Input: part model. Units: mm. Frame: model coordinates. A direction names the side the tool comes from. Coordinates: 2 decimals unless noted, no trailing zeros. Write each loop counter-clockwise with the first axis right and the second up, starting at its lowest first coordinate (ties: lowest second). Pieces come first, ordered by that corner, then holes. Notation, with made-up numbers: (-2.5, 38.25) - (15.5, 38.25) arc R3 cw to (15.5, 43.25) - close; hole circle Ø7 at (45, -20). An arc over 180 degrees is marked (long way). Put each result on its own line as item: value. Start each with the question number.
1. Cut plane A-A, the plane z = -32. Return loops of the section in (x, y), and give its area (3 significant figures).
2. Access query for faces 4 (the cylindrical face through (-8, -48, -8)), 5 (the flat face through (-153, 5, -58)), 6 (the flat face through (-200, 2, -61)), 7 (the cylindrical face through (-101, -48, -64)). Directions: +Z, -Z, +X, -X, +Y, -Y. A direction counts if a zero-diameter tool reaches every point of the face in a straight line with its end or side. Return the directions, or none.
3. Line query: line 1 (X direction, y = 2, z = -4); line 2 (X direction, y = 3, z = -62); line 3 (Z direction, x = -189, y = -51). Output: solid intervals per line, ascending.
4. Pull-direction query (Z, two-part tool) for faces 1 (the flat face through (-110, 3, -27)), 2 (the flat face through (-97, -27, -67)), 3 (the flat face through (-197, 4.5, -61)); classes: released by +Z, released by -Z, zero draft, split by the parting line, or undercut.
5. Cut plane C-C, the plane x = -164. Return loops of the section in (y, z), and give its area (3 significant figures).
6. Pin query (flat end, axial travel): pin 1 (1.5 mm diameter, centred on y = -27, z = -65, fed in from +X); pin 2 (2 mm diameter, centred on y = 4.5, z = -36.5, fed in from -X); pin 3 (3.5 mm diameter, centred on x = -178.5, y = 1.5, fed in from +Z); pin 4 (1.5 mm diameter, centred on y = -6.5, z = -67.5, fed in from -X). Return the tip coordinate at first contact, or that it passes through.
7. Cut plane B-B, the plane y = -48. Return loops of the section in (x, z), and give its area (3 significant figures).
Autodesk Inventor part; units mm, degrees
ref_plane "YZ Plane" through (0, 0, 0) normal (1, 0, 0) x (0, 1, 0)
ref_plane "XZ Plane" through (0, 0, 0) normal (0, 1, 0) x (-1, 0, 0)
ref_plane "XY Plane" through (0, 0, 0) normal (0, 0, 1) x (1, 0, 0)
sketch "スケッチ1" plane through (0, 0, 0) normal (0, 1, 0) x (-1, 0, 0)
  line L0 (0, 0) -> (204, 0)
  line L1 (204, 0) -> (204, -72)
  line L2 (204, -72) -> (0, -72)
  line L3 (0, -72) -> (0, 0)
  dimension "d0" = 204
  dimension "d1" = 72
extrude "押し出し1" add sketch "スケッチ1" along normal blind 7
sketch "スケッチ2" plane through (0, 7, 0) normal (0, 1, 0) x (1, 0, 0)
  line L0 (-204, 72) -> (-204, 0)
  line L1 (-204, 0) -> (-112, 0)
  line L2 (-112, 0) -> (-112, 50)
  line L3 (-112, 50) -> (-204, 50)
  line L4 (-204, 50) -> (-204, 0)
  point P0 (0, 0)
  dimension "d4" = 92
  dimension "d5" = 50
extrude "押し出し2" cut sketch "スケッチ2" against normal through all
sketch "スケッチ3" plane through (0, 7, 0) normal (0, 1, 0) x (1, 0, 0)
  line L0 (-112, 0) -> (0, 0)
  line L1 (0, 0) -> (0, 72)
  line L2 (-112, 0) -> (0, 0)
  line L3 (0, 0) -> (0, 8)
  line L4 (0, 8) -> (-112, 8)
  line L5 (-112, 8) -> (-112, 0)
  line L6 (-112, 0) -> (-104, 0)
  line L7 (-104, 0) -> (-104, 58)
  line L8 (-104, 58) -> (-112, 58)
  line L9 (-112, 58) -> (-112, 0)
  line L10 (-204, 72) -> (-204, 50)
  line L11 (-204, 50) -> (-104, 50)
  line L12 (-104, 50) -> (-104, 58)
  line L13 (-104, 58) -> (-204, 58)
  line L14 (-204, 58) -> (-204, 50)
  point P0 (-112, 50)
  point P1 (-112, 8)
  point P2 (-104, 8)
  dimension "d8" = 8
  dimension "d11" = 8
  dimension "d12" = 8
extrude "押し出し3" cut sketch "スケッチ3" against normal blind 4
sketch "スケッチ4" plane through (0, 3, 0) normal (0, 1, 0) x (1, 0, 0)
  circle A0 centre (-192, 54) radius 1.5
  circle A1 centre (-108, 54) radius 1.5
  circle A2 centre (-108, 13) radius 1.5
  circle A3 centre (-12, 4) radius 1.5
  circle A4 centre (-88, 4) radius 1.5
  line L0 (-204, 50) -> (-204, 58)
  line L1 (0, 8) -> (0, 0)
  line L2 (-112, 0) -> (-112, 50)
  point P0 (-204, 54)
  point P1 (-204, 54)
  point P2 (0, 4)
  point P3 (0, 4)
  dimension "d13" = 3
  dimension "d14" = 3
  dimension "d15" = 3
  dimension "d16" = 3
  dimension "d17" = 3
  dimension "d18" = 12
  dimension "d19" = 12
  dimension "d20" = 24
  dimension "d21" = 4
  dimension "d22" = 41
extrude "押し出し4" cut sketch "スケッチ4" against normal through all
sketch "スケッチ5" plane through (0, 0, 0) normal (0, -1, 0) x (1, 0, 0)
  line L0 (-112, -50) -> (-204, -50)
  line L1 (0, -72) -> (-204, -72)
  line L2 (-204, -50) -> (-196, -50)
  line L3 (-196, -50) -> (-196, -72)
  line L4 (-196, -72) -> (-204, -72)
  line L5 (-204, -72) -> (-204, -50)
  point P0 (0, 0)
  point P1 (-204, -72)
  dimension "d25" = 8
extrude "押し出し5" cut sketch "スケッチ5" against normal blind 2
sketch "スケッチ6" plane through (0, 0, 0) normal (0, -1, 0) x (1, 0, 0)
  line L0 (0, -72) -> (-204, -72)
  line L1 (-196, -50) -> (-196, -72)
  line L2 (0, -72) -> (-196, -72)
  line L3 (-196, -72) -> (-196, -67)
  line L4 (-196, -67) -> (0, -67)
  line L5 (0, -67) -> (0, -72)
  line L6 (0, 0) -> (-5, 0)
  line L7 (-5, 0) -> (-5, -72)
  line L8 (-5, -72) -> (0, -72)
  line L9 (0, -72) -> (0, 0)
  point P0 (-5, -67)
  dimension "d28" = 5
  dimension "d29" = 5
extrude "押し出し6" add sketch "スケッチ6" along normal blind 55
sketch "スケッチ7" plane through (-196, 0, -67) normal (0, 0, 1) x (1, 0, 0)
  line L0 (0, 2) -> (0, -55)
  line L1 (0, 0) -> (191, 0)
  line L2 (0, -55) -> (10, -55)
  line L3 (10, -55) -> (10, 0)
  line L4 (10, 0) -> (0, 0)
  line L5 (0, 0) -> (0, -55)
  point P0 (196, 0)
  dimension "d32" = 10
extrude "押し出し7" add sketch "スケッチ7" along normal blind 3
sketch "スケッチ8" plane through (-196, 2, -72) normal (-1, 0, 0) x (0, 0, 1)
  circle A0 centre (4, -41) radius 1.5
  circle A1 centre (4, -8) radius 1.5
  line L0 (0, -57) -> (8, -57)
  line L1 (0, 0) -> (22, 0)
  point P0 (72, -2)
  point P1 (4, -57)
  point P2 (4, -57)
  point P3 (4, -57)
  dimension "d35" = 3
  dimension "d36" = 3
  dimension "d37" = 16
  dimension "d38" = 8
extrude "押し出し8" cut sketch "スケッチ8" against normal blind 8
sketch "スケッチ9" plane through (0, -55, 0) normal (0, -1, 0) x (1, 0, 0)
  line L0 (-5, -67) -> (-5, 0)
  circle A0 centre (-5, -8) radius 3
  circle A1 centre (-5, -67) radius 3
  line L1 (-186, -67) -> (-5, -67)
  circle A2 centre (-101, -67) radius 3
  circle A3 centre (-191, -67) radius 3
  line L2 (0, 0) -> (-5, 0)
  dimension "d41" = 6
  dimension "d42" = 6
  dimension "d43" = 6
  dimension "d44" = 6
  dimension "d46" = 96
  dimension "d47" = 90
  dimension "d73" = 8
extrude "押し出し9" add sketch "スケッチ9" against normal blind 15
sketch "スケッチ10" plane through (0, -55, 0) normal (0, -1, 0) x (1, 0, 0)
  arc A0 (-5, -5) -> (-5, -11) centre (-5, -8) ccw
  circle A1 centre (-5, -8) radius 1.5
  arc A2 (-5, -64) -> (-8, -67) centre (-5, -67) ccw
  circle A3 centre (-5, -67) radius 1.5
  arc A4 (-98, -67) -> (-104, -67) centre (-101, -67) ccw
  circle A5 centre (-101, -67) radius 1.5
  circle A6 centre (-189, -67) radius 1.5
  line L0 (-186, -67) -> (-186, -64)
  line L1 (-196, -64) -> (-186, -64)
  dimension "d50" = 3
  dimension "d51" = 3
  dimension "d52" = 3
  dimension "d58" = 3
  dimension "d59" = 3
  dimension "d60" = 3
extrude "押し出し10" cut sketch "スケッチ10" against normal blind 12
sketch "スケッチ11" plane through (0, 7, 0) normal (0, 1, 0) x (1, 0, 0)
  circle A0 centre (-198.5, 62) radius 1.5
  line L0 (-204, 72) -> (-204, 58)
  line L1 (0, 72) -> (-204, 72)
  line L2 (-204, 58) -> (-104, 58)
  point P0 (0, 0)
  dimension "d61" = 3
  dimension "d63" = 5.5
  dimension "d75" = 4
extrude "押し出し11" cut sketch "スケッチ11" against normal through all
sketch "スケッチ12" plane through (0, 7, 0) normal (0, 1, 0) x (1, 0, 0)
  circle A0 centre (-198.5, 62) radius 2.8
  circle A1 centre (-198.5, 62) radius 1.5
  point P0 (0, 0)
  dimension "d68" = 5.6
extrude "押し出し12" cut sketch "スケッチ12" against normal blind 2.5 contours A0 | A1
fillet "フィレット1" radius 2 4 edges at (-204, 7, -65) (-102, 7, -72) (0, 7, -40) (0, -24, -72)
properties part number "オンゲキボタン_top_right2_3D プリント"
Report:
1. outline: (-112, 0) - (-5, 0) - (-5, -55) - (0, -55) - (0, 5) arc R2 ccw to (-2, 7) - (-104, 7) - (-104, 3) - (-112, 3) - close
1. area: 1,030 mm^2
2. face 4: -X, -Y
2. face 5: +Z, -X, +Y
2. face 6: +Z, -Z, -X, -Y
2. face 7: +Z, -Y
3. line 1: x = -112 to -89.5, -86.5 to -13.5, -10.5 to 0
3. line 2: x = -204 to -200, -197 to 0
3. line 3: z = -72 to -68.5, -65.5 to -64
4. face 1: zero draft
4. face 2: released by +Z
4. face 3: undercut
5. outline: (-55, -72) - (5, -72) arc R2 ccw to (7, -70) - (7, -58) - (3, -58) - (3, -50) - (0, -50) - (0, -67) - (-55, -67) - close
5. area: 396 mm^2
6. pin 1: stops at x = 0
6. pin 2: stops at x = -104
6. pin 3: stops at z = -50
6. pin 4: stops at x = -188
7. outline: (-196, -72) - (-2, -72) arc R2 ccw to (0, -70) - (0, 0) - (-5, 0) - (-5, -5) arc R3 ccw to (-5, -11) - (-5, -64) arc R3 ccw to (-8, -67) - (-98, -67) arc R3 ccw to (-104, -67) - (-186, -67) - (-186, -64) - (-196, -64) - close; hole circle Ø3 at (-189, -67); hole circle Ø3 at (-101, -67); hole circle Ø3 at (-5, -67); hole circle Ø3 at (-5, -8)
7. area: 1,350 mm^2
